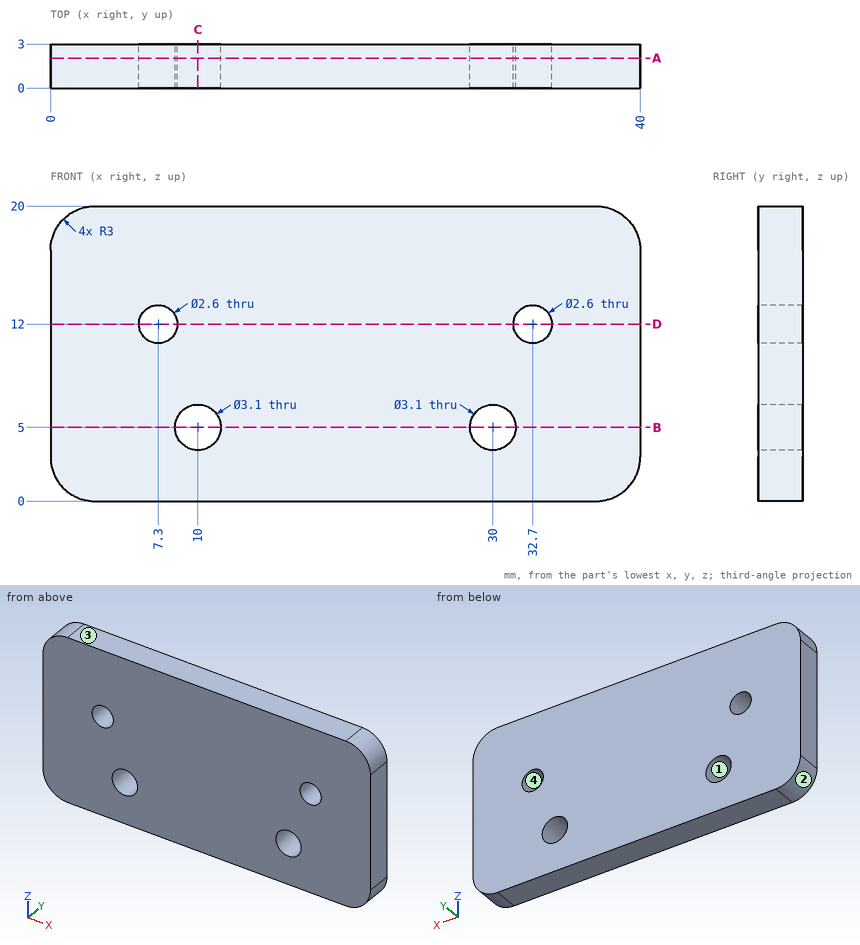
Print and shaded views of the part. All mm, measured from the part's lowest x, y and z. Coordinates: 2 decimals unless noted, no trailing zeros. Loops run counter-clockwise (first coordinate to the right, second up) from the corner with the lowest first, then second, coordinate; pieces in that order, holes last. Notation, with made-up numbers: (1, 57) - (7, 57) arc R31 ccw to (7, 91) - close; hole circle Ø11 at (-26, -6.5). An arc over 180 degrees is marked (long way). Use one line per item in the form item = value. Start each with the question number.
1) Band-saw the part on D-D (z = 12). Give the cut face in (x, y).
2) Two-plate mould, pull along X, no slides. Class the marked faces 1, 2, 3 and 4: +X half, -X half, draft (parallel to the pull), parting line (faces both ways), or undercut.
3) Band-saw the part on B-B (z = 5). Give the cut face in (x, y), and give its area (3 significant figures).
4) Band-saw the part on A-A (y = 2.05). Give the cut face in (x, z).
5) Band-saw the part on C-C (x = 10). Give the cut face in (y, z).
6) Drill centre lines: L1, parallel to X at y = 0.75, z = 5; L2, parallel to X at y = 0.25, z = 4; L3, parallel to Z at x = 30, y = 1.6. Where is each one in solid material? Low to high. Write a range as from..to.
Check values:
q1.outline = (0, 0) - (6, 0) - (6, 3) - (0, 3) - close; (8.6, 0) - (31.4, 0) - (31.4, 3) - (8.6, 3) - close; (34, 0) - (40, 0) - (40, 3) - (34, 3) - close
q2.face_1 = undercut
q2.face_2 = -X half
q2.face_3 = draft
q2.face_4 = undercut
q3.outline = (0, 0) - (8.45, 0) - (8.45, 3) - (0, 3) - close; (11.55, 0) - (28.45, 0) - (28.45, 3) - (11.55, 3) - close; (31.55, 0) - (40, 0) - (40, 3) - (31.55, 3) - close
q3.area = 101 mm2
q4.outline = (0, 3) arc R3 ccw to (3, 0) - (37, 0) arc R3 ccw to (40, 3) - (40, 17) arc R3 ccw to (37, 20) - (3, 20) arc R3 ccw to (0, 17) - close; hole circle Ø2.6 at (7.3, 12); hole circle Ø3.1 at (10, 5); hole circle Ø3.1 at (30, 5); hole circle Ø2.6 at (32.7, 12)
q5.outline = (0, 0) - (3, 0) - (3, 3.45) - (0, 3.45) - close; (0, 6.55) - (3, 6.55) - (3, 20) - (0, 20) - close
q6.L1 = 0..8.45, 11.55..28.45, 31.55..40
q6.L2 = 0..8.82, 11.18..28.82, 31.18..40
q6.L3 = 0..3.45, 6.55..20
